For this review, use the dimensioned drawing (mm, ordinates from the lowest corner) and the shaded views. A direction names the side the tool comes from. Give positions to 0.01 mm unless a question says otherwise; leave off trailing zeros. Loops run counter-clockwise (first coordinate to the right, second up) from the corner with the lowest first, then second, coordinate; pieces in that order, holes last. Notation, with made-up numbers: M 72.5,-18.5 L 91.5,-18.5 A23 ccw 91.5,1.5 Z; hole C 63.25,32 d11. An arc over 180 degrees is marked long. Use CSV: the item, a comma, the result in double quotes.
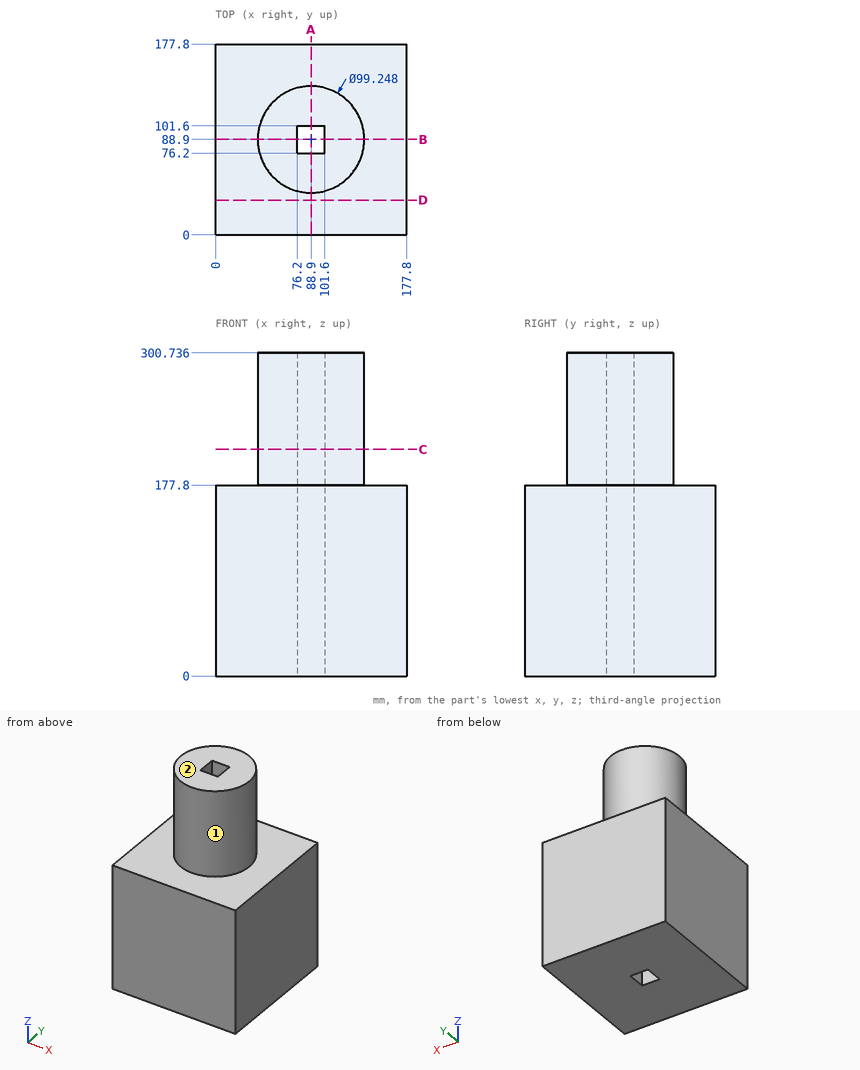
(1) We need section C-C on z = 211. State the section outline as (x, y) points, then the cut area to 3 significant figures.
A:
outline,"C 88.9,88.9 d99.25; hole M 76.2,76.2 L 101.6,76.2 L 101.6,101.6 L 76.2,101.6 Z"
area,"7,090 mm²"
(2) Clearance check with flat-ended pins moving along their axes: P1, Ø3, axis at x = 133, y = 26.5, coming from the +Z side; P2, Ø7.5, axis at x = 94, z = 220, coming from the -Y side; P3, Ø1.5, axis at x = 104, z = 221.5, coming from the -Y side. State where each tip first meets the part, or that it passes through.
A:
P1,"z = 177.8"
P2,"y = 39.29"
P3,"y = 41.4"
(3) Machinability: for the marked faces 1 and 2, which of the approach directions +Z, -Z, +X, -X, +Y, -Y give a long, thin tool a straight path to every point of the face, cutting with its end or side? Answer none if there is none.
A:
face 1,"+Z"
face 2,"+Z, +X, -X, +Y, -Y"
(4) We need section A-A on x = 88.9. State the section outline as (y, z) points.
A:
outline,"M 0,0 L 76.2,0 L 76.2,300.74 L 39.28,300.74 L 39.28,177.8 L 0,177.8 Z; M 101.6,0 L 177.8,0 L 177.8,177.8 L 138.52,177.8 L 138.52,300.74 L 101.6,300.74 Z"
(5) Wall thickness on line 1 along Y through (x, z) = (98.5, 57); line 2 along Z through (x, y) = (70, 158); line 3 along Y through (x, z) = (86, 273): over which ranges is each line inside the solid? List them lowest first. Write a range as [from, to].
A:
line 1,"[0, 76.2], [101.6, 177.8]"
line 2,"[0, 177.8]"
line 3,"[39.36, 76.2], [101.6, 138.44]"
(6) We need section D-D on y = 32.5. State the section outline as (x, z) points, then the cut area to 3 significant figures.
A:
outline,"M 0,0 L 177.8,0 L 177.8,177.8 L 0,177.8 Z"
area,"31,600 mm²"
